Geometry: see drawing. Coordinates: mm, zero at the bounding-box minimum. A direction names the side the tool comes from. Give positions to 0.01 mm unless a question says otherwise; leave off trailing zeros. Loops run counter-clockwise (first coordinate to the right, second up) from the corner with the lowest first, then second, coordinate; pieces in that order, holes last. Notation, with made-up numbers: (0.5, 48.25) - (25.5, 48.25) arc R22 cw to (25.5, 85.25) - close; hole circle Ø5 at (-8, -34). An arc over 180 degrees is marked (long way). Use CSV: the item, a comma, the result in double quotes. Start each with the question number.
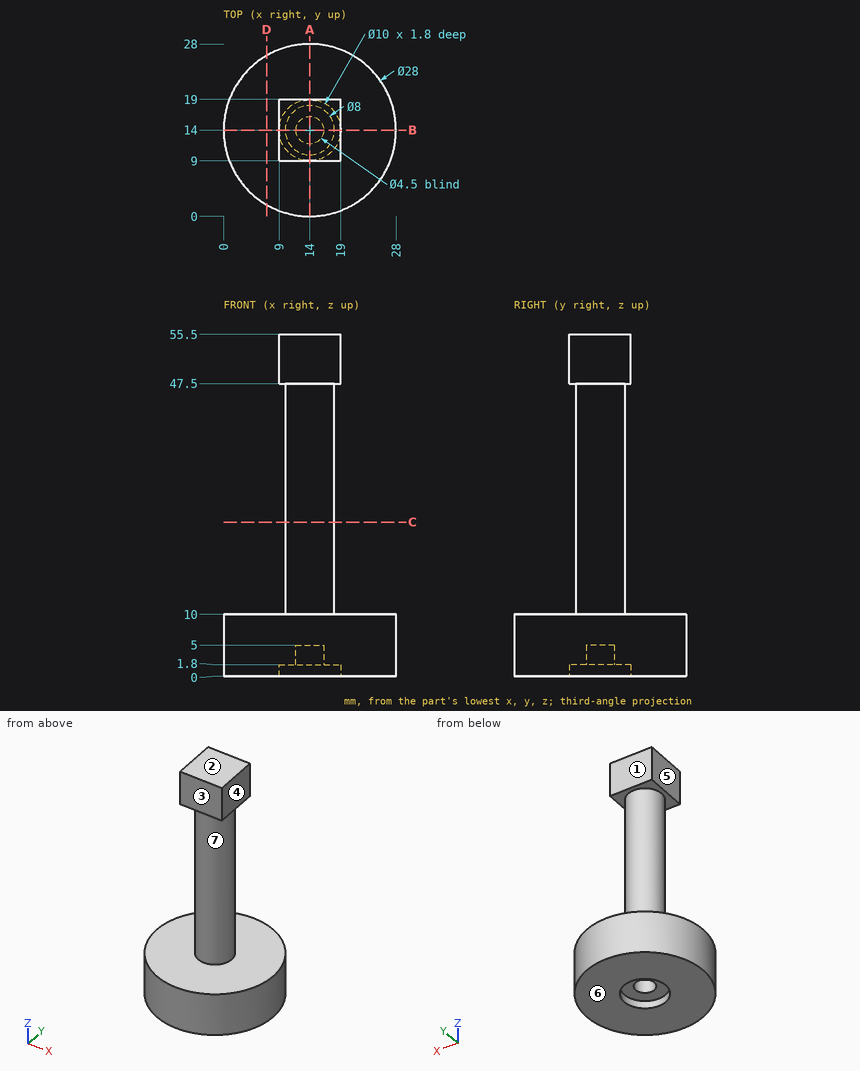
Item 1: Pin query (flat end, axial travel): pin 1 Ø1.5 at (y, z) = (16, 6) entering from -X; pin 2 Ø6.5 at (y, z) = (14.5, 50) entering from +X; pin 3 Ø9 at (x, z) = (14.5, 49.5) entering from +Y. Return the tip coordinate at first contact, or that it passes through.
Item 2: Section C-C (z = 25). Output: boundary loops of the cut face in (x, y), plus the area to 3 significant figures.
Item 3: Mould query, pull axis Z, two halves, no side actions, for the marked faces 5, 6 and 7. Classes: pulls with the +Z half, pulls with the -Z half, needs draft (parallel to the pull), parting line crosses it, or undercut.
Item 4: Reachability of the marked faces 1, 2, 3 and 4 from +Z, -Z, +X, -X, +Y, -Y: full face, straight path, thin tool, end or side. Return the list, or none.
Item 5: Section D-D (x = 7). Output: boundary loops of the cut face in (y, z).
Item 6: Section A-A (x = 14). Output: boundary loops of the cut face in (y, z), plus the area to 3 significant figures.
Item 7: Ray query, probe 1 along Y at (x, z) = (14, 0.85); probe 2 along Z at (x, y) = (18, 16.25); probe 3 along Y at (x, z) = (14, 2.5). Return the intervals inside material, ascending.
Outcome:
1,pin 1,"stops at x = 0.06"
1,pin 2,"stops at x = 19"
1,pin 3,"stops at y = 19"
2,outline,"circle Ø8 at (14, 14)"
2,area,"50.3 mm2"
3,face 5,"needs draft"
3,face 6,"pulls with the -Z half"
3,face 7,"undercut"
4,face 1,"+Z, +X, -X, +Y"
4,face 2,"+Z, +X, -X, +Y, -Y"
4,face 3,"+Z, +X, -X, -Y"
4,face 4,"+Z, +X, +Y, -Y"
5,outline,"(1.88, 0) - (26.12, 0) - (26.12, 10) - (1.88, 10) - close"
6,outline,"(0, 0) - (9, 0) - (9, 1.8) - (11.75, 1.8) - (11.75, 5) - (16.25, 5) - (16.25, 1.8) - (19, 1.8) - (19, 0) - (28, 0) - (28, 10) - (18, 10) - (18, 47.5) - (19, 47.5) - (19, 55.5) - (9, 55.5) - (9, 47.5) - (10, 47.5) - (10, 10) - (0, 10) - close"
6,area,"628 mm2"
7,probe 1,"y = 0 to 9, 19 to 28"
7,probe 2,"z = 1.8 to 10, 47.5 to 55.5"
7,probe 3,"y = 0 to 11.75, 16.25 to 28"
